```python
from build123d import *

# Parameters (mm, degrees)
F1_DEPTH = 19.05
F2_W     = 3.175
F2_H     = 9.6882774726
F3_DEPTH = 12.7


# Not quite as in the source:
# - ends of sketch curves that miss each other by under 0.0002 mm in the source are joined


with BuildPart() as f1:
    # F0 (on Front) → F1 (new body)
    with BuildSketch(Plane.XZ):
        Polygon((-7.493, 0.1328983575), (0, 0.1328983575), (7.493, 0.1328983575), (22.2194990303, 0.1328983575), (22.2194990303, 19.5094533027), (7.7658264293, 31.8828983575), (7.7658264293, 38.2328983575), (-7.7713273633, 38.2328983575), (-7.7713273633, 31.8828983575), (-22.2249999642, 19.5094533027), (-22.2249999642, 4.5234533027), (-22.2249999642, 0.1328983575), align=None)
        with BuildLine():
            ThreePointArc((-1.6471995105, 13.7654938087), (-14.0416307026, 9.056743723), (-13.4701421127, 22.3031640975))
            Line((-13.4701421127, 22.3031640975), (-7.8430329322, 27.1203983575))
            Line((-7.8430329322, 27.1203983575), (-3.175, 27.1203983575))
            Line((-3.175, 27.1203983575), (-3.175, 30.2953983575))
            Line((-3.175, 30.2953983575), (-3.175, 33.4703983575))
            Line((-3.175, 33.4703983575), (3.175, 33.4703983575))
            Line((3.175, 33.4703983575), (3.175, 30.2953983575))
            Line((3.175, 30.2953983575), (3.175, 27.1203983575))
            Line((3.175, 27.1203983575), (7.8375319983, 27.1203983575))
            Line((7.8375319983, 27.1203983575), (13.4701421127, 22.3031640975))
            ThreePointArc((13.4701421127, 22.3031640975), (16.2995077669, 19.40684068), (17.3322006389, 15.4917998403))
            ThreePointArc((17.3322006389, 15.4917998403), (10.2711150187, 7.6028326022), (1.6507381924, 13.7496885133))
            ThreePointArc((1.6507381924, 13.7496885133), (0.0063534061, 14.7141035739), (-1.6471995105, 13.7654938087))
        make_face(mode=Mode.SUBTRACT)
    extrude(amount=F1_DEPTH)

    # F2 (on face) → F3 (join)
    with BuildSketch(Plane(origin=(0, 0, 0), x_dir=(-1, 0, 0), z_dir=(0, 1, 0))):
        with Locations((-20.6319990303, 14.6653145664)):
            Rectangle(F2_W, F2_H)
        with Locations((20.6374999642, 14.6653145664)):
            Rectangle(F2_W, F2_H)
        Polygon((-4.239049533, 3.3078983575), (-4.239049533, 0.1328983575), (0.002750467, 0.1328983575), (4.244550467, 0.1328983575), (4.244550467, 3.3078983575), align=None)
    extrude(amount=F3_DEPTH)


solid = f1.part
```
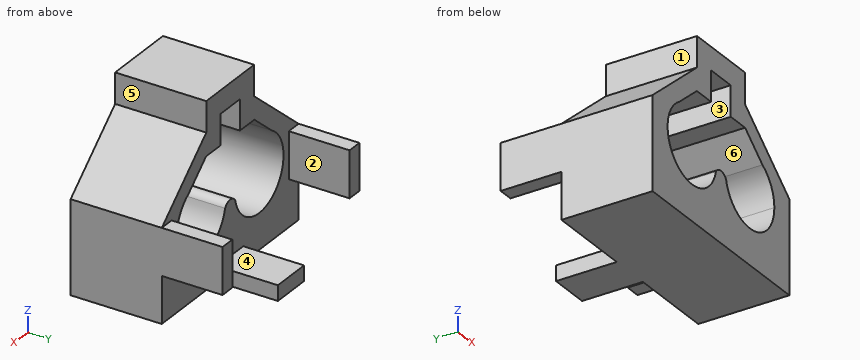
For this review, take the finished solid that the model builds, in its own axes (mm). Face numbers are marked on the shaded views. A direction names the side the tool comes from. Coordinates: 2 decimals unless noted, no trailing zeros. Order: outer loops, then holes, each group sorted by start corner. A loop starts at its lowest first (then second) coordinate and runs counter-clockwise, first axis right, second up. Notation, with made-up numbers: (-7.5, 58.5) - (48.5, 58.5) arc R18 cw to (48.5, 70.5) - close; hole circle Ø10 at (21, 35.25). An arc over 180 degrees is marked (long way). Answer as a JSON object with one key per item and string values. Group by question number.
1. We need section A-A on y = 7.5. Give the number of separate pieces and of enclosed holes in the cut face, then the cut area to 3 significant figures.
2. For probe 1 along X at (y, z) = (-14, 14) (1 decimal); probe 2 along X at (y, z) = (-1, 32) (3 decimals); probe 3 along Y at (x, z) = (8, 28), list the stretches that pass through material, from the lowest coordinate up.
3. The part is to be moulded in two halves that separate along Z. For the marked faces 4, 5 and 6, say which applies: pulls with the +Z half, pulls with the -Z half, needs draft (parallel to the pull), parting line crosses it, or undercut.
4. Clearance check with flat-ended pins moving along their axes: P1, Ø19, axis at x = 1.5, z = 18, coming from the +Y side; P2, Ø2, axis at y = -9.5, z = 30, coming from the +X side; P3, Ø1.6, axis at y = 9, z = 2.5, coming from the +X side; P4, Ø4, axis at x = 8, z = 22.5, coming from the +Y side. State where each tip first meets the part, or that it passes through.
5. We need section C-C on y = -9. State the section outline as (x, z) points (1 decimal).
6. For the marked faces 1, 2 and 3, list the 3-axis set-ups (+Z, -Z, +X, -X, +Y, -Y) from which the entire face can be reached by the end or side of a thin tool; tool diameter is ignored.
7. We need section B-B on x = 11.5. State the section outline as (y, z) points, then the cut area to 3 significant figures.
8. We need section D-D on x = 5. State the section outline as (y, z) points.
Final values:
{
 "1": {"separate pieces": "3", "enclosed holes": "0", "area": "88.5 mm²"},
 "2": {"probe 1": "-22.2 to -17.2, -1.5 to 1.5, 17.2 to 22.2", "probe 2": "-7.771 to -3.175, 3.175 to 7.766", "probe 3": "-19.05 to 0"},
 "3": {"face 4": "pulls with the +Z half", "face 5": "needs draft", "face 6": "undercut"},
 "4": {"P1": "y = 0", "P2": "x = 11.13", "P3": "x = 4.24", "P4": "through"},
 "5": {"outline": "(-22.2, 0.1) - (22.2, 0.1) - (22.2, 19.5) - (7.8, 31.9) - (7.8, 38.2) - (-7.8, 38.2) - (-7.8, 31.9) - (-22.2, 19.5) - close; hole (-13.5, 22.3) arc R7.9 ccw (long way) to (-1.6, 13.8) arc R1.9 cw to (1.7, 13.7) arc R7.9 ccw (long way) to (13.5, 22.3) - (7.8, 27.1) - (3.2, 27.1) - (3.2, 33.5) - (-3.2, 33.5) - (-3.2, 27.1) - (-7.8, 27.1) - close"},
 "6": {"face 1": "+Z, -X, +Y, -Y", "face 2": "+Z, -Z, +Y", "face 3": "+Y, -Y"},
 "7": {"outline": "(-19.05, 0.13) - (0, 0.13) - (0, 7.84) - (-19.05, 7.84) - close; (-19.05, 23.99) - (0, 23.99) - (0, 28.69) - (-19.05, 28.69) - close", "area": "236 mm²"},
 "8": {"outline": "(-19.05, 0.13) - (0, 0.13) - (0, 8.88) - (-19.05, 8.88) - close; (-19.05, 27.12) - (0, 27.12) - (0, 38.23) - (-19.05, 38.23) - close"}
}
